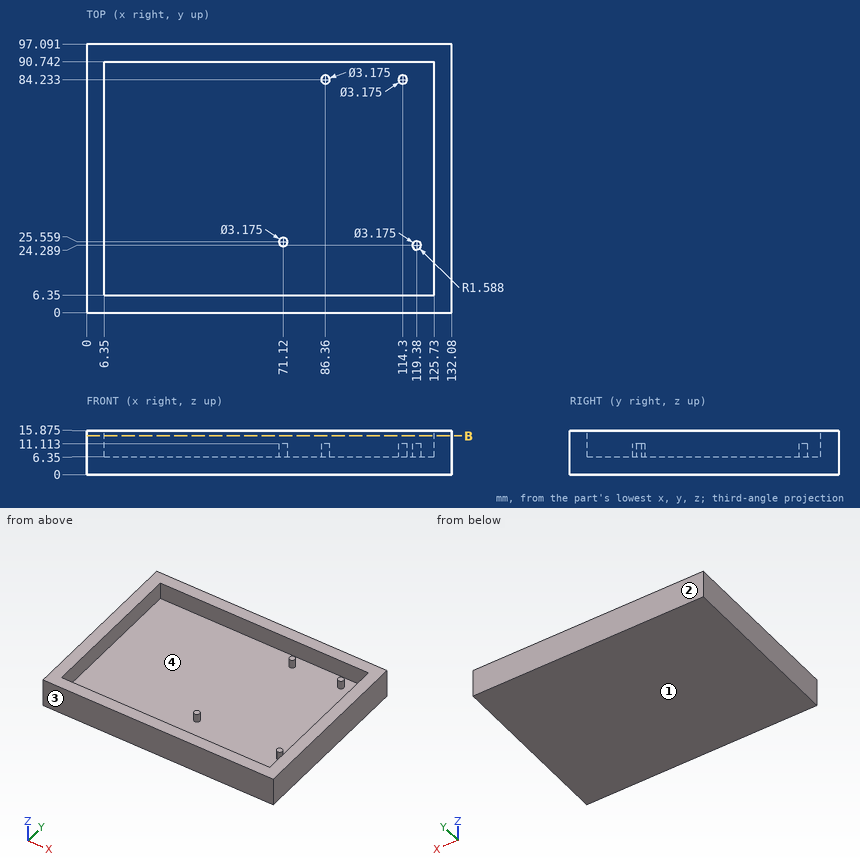
Verification items for this drawing (mm, ordinates from the low corner). Coordinates: 2 decimals unless noted, no trailing zeros. Loops run counter-clockwise (first coordinate to the right, second up) from the corner with the lowest first, then second, coordinate; pieces in that order, holes last.
Item 1: Release check for a two-part mould opening along Y. For the marked faces 1, 2, 3 and 4 record: released by +Y, released by -Y, zero draft, split by the parting line, or undercut.
Item 2: Thickness scan on line 1 (Y direction, x = 34.5, z = 11.5); line 2 (X direction, y = 35.5, z = 14); line 3 (Z direction, x = 114, y = 55). Record the ranges inside material, lowest first.
Item 3: Go/stop test with flat-tipped pins: pin 1 Ø1 at (x, y) = (119, 23.5) entering from +Z; pin 2 Ø6 at (y, z) = (17, 7) entering from -X; pin 3 Ø6 at (x, y) = (81, 10) entering from +Z. Record where each tip stops, or that it passes through.
Item 4: Sectioned sample at B-B, the plane z = 14. Record the boundary of the cut face in (x, y), then the cut area to 3 significant figures.
Check result:
1. face 1: zero draft
1. face 2: released by +Y
1. face 3: released by -Y
1. face 4: undercut
2. line 1: y = 0 to 6.35, 90.74 to 97.09
2. line 2: x = 0 to 6.35, 125.73 to 132.08
2. line 3: z = 0 to 6.35
3. pin 1: stops at z = 11.11
3. pin 2: stops at x = 0
3. pin 3: stops at z = 6.35
4. outline: (0, 0) - (132.08, 0) - (132.08, 97.09) - (0, 97.09) - close; hole (6.35, 6.35) - (125.73, 6.35) - (125.73, 90.74) - (6.35, 90.74) - close
4. area: 2,750 mm2
